The listing builds one solid part. Answer for the finished solid, in the listing's coordinates (mm). Give positions to 0.01 mm unless a question says otherwise; leave off trailing zeros. Write each loop counter-clockwise with the first axis right and the second up, starting at its lowest first coordinate (ties: lowest second). Pieces come first, ordered by that corner, then holes. Notation, with made-up numbers: M 57,-35 L 63,-35 A23 cw 63,-7 Z; hole C -27.75,57.5 d3. An arc over 180 degrees is marked long. Answer as a JSON object with one key per item and string values.
Autodesk Inventor part; units mm, degrees
ref_plane "YZ Plane" through (0, 0, 0) normal (1, 0, 0) x (0, 1, 0)
ref_plane "XZ Plane" through (0, 0, 0) normal (0, 1, 0) x (-1, 0, 0)
ref_plane "XY Plane" through (0, 0, 0) normal (0, 0, 1) x (1, 0, 0)
sketch "Sketch1" plane through (0, 0, 0) normal (0, 1, 0) x (-1, 0, 0)
  circle A0 centre (0, 0) radius 16.575
  circle A1 centre (0, 0) radius 2.5
  dimension "d0" = 33.15
  dimension "d1" = 5
extrude "Extrusion1" add sketch "Sketch1" along normal blind 3.8
sketch "Sketch2" plane through (0, 3.8, 0) normal (0, 1, 0) x (1, 0, 0)
  circle A0 centre (0, 0) radius 2.5
  circle A1 centre (0, 0) radius 16.575
  line L0 (-2.5, 0) -> (-16.575, 0)
  circle A2 centre (-9.5375, 0) radius 1.5
  line L1 (0, 0) -> (16.575, 0) construction
  line L2 (0, 0) -> (16.575, 0) construction
  circle A3 centre (4.7688, 8.2597) radius 1.5
  circle A4 centre (4.7688, -8.2597) radius 1.5
  dimension "d4" = 3
  dimension "d7" = 3
  dimension "d8" = 3
extrude "Extrusion2" cut sketch "Sketch2" against normal blind 3.8 contours A2 L0 | L0 A2 | A3 | A4
sketch "Sketch3" plane through (0, 0, 0) normal (0, -1, 0) x (1, 0, 0)
  circle A0 centre (4.7688, -8.2597) radius 1.5
  circle A1 centre (-9.5375, 0) radius 1.5
  circle A2 centre (4.7688, 8.2597) radius 1.5
  circle A3 centre (-9.5375, 0) radius 1
  circle A4 centre (4.7688, 8.2597) radius 1
  circle A5 centre (4.7688, -8.2597) radius 1
  dimension "d11" = 2
  dimension "d12" = 2
  dimension "d13" = 2
extrude "Extrusion3" add sketch "Sketch3" against normal blind 3.8
properties part number "kolecko_rameno(3)"
1. The mould has two halves that part along X. Classify faces 1 (the cylindrical face through (-10.537, 1.873, 0.044)), 2 (the cylindrical face through (4.64, 1.87, -7.27)), 3 (the flat face through (0, 3.8, -3)), 4 (the cylindrical face through (3.59, 1.87, 16.18)): released by +X, released by -X, zero draft, split by the parting line, or undercut.
Verdict:
{"face 1": "undercut", "face 2": "undercut", "face 3": "zero draft", "face 4": "split by the parting line"}
2. A cutting plane is placed at A-A, the plane z = 0. Give the vertices of the cut face in (x, y) (1 decimal).
Verdict:
{"outline": "M -16.6,0 L -10.5,0 L -10.5,3.8 L -16.6,3.8 Z; M -8.5,0 L -2.5,0 L -2.5,3.8 L -8.5,3.8 Z; M 2.5,0 L 16.6,0 L 16.6,3.8 L 2.5,3.8 Z"}
3. A cutting plane is placed at C-C, the plane y = 3.05. Count the separate pieces of the cut face and the enclosed holes in it, plus the area to 3 significant figures.
Verdict:
{"separate pieces": "1", "enclosed holes": "4", "area": "834 mm2"}
4. Consider line 1 along Z through (x, y) = (0, 2.5) (3 decimals); line 2 along Z through (x, y) = (4, 1.1); line 3 along Z through (x, y) = (-2, 1.8). Determine where each line is inside the solid, lowest interval first.
Verdict:
{"line 1": "z = -16.575 to -2.5, 2.5 to 16.575", "line 2": "z = -16.09 to -8.9, -7.62 to 7.62, 8.9 to 16.09", "line 3": "z = -16.45 to -1.5, 1.5 to 16.45"}
5. Flat-ended cylindrical pins translate along their axes: pin 1 (1.5 mm diameter, centred on y = 1, z = 8, fed in from -X); pin 2 (1.8 mm diameter, centred on x = 4.77, z = 8.26, fed in from +Y). Find the tip coordinate at first contact, or state that the pin passes through.
Verdict:
{"pin 1": "stops at x = -14.91", "pin 2": "passes through"}
6. A cutting plane is placed at B-B, the plane x = 0. Give the vertices of the cut face in (y, z) (3 decimals), plus the area to 3 significant figures.
Verdict:
{"outline": "M 0,-16.575 L 3.8,-16.575 L 3.8,-2.5 L 0,-2.5 Z; M 0,2.5 L 3.8,2.5 L 3.8,16.575 L 0,16.575 Z", "area": "107 mm2"}
7. A cutting plane is placed at D-D, the plane x = -6. Give the vertices of the cut face in (y, z).
Verdict:
{"outline": "M 0,-15.45 L 3.8,-15.45 L 3.8,15.45 L 0,15.45 Z"}
